Could you check a few things on this model? Use its own coordinates, in mm. Coordinates: 2 decimals unless noted, no trailing zeros. Loops run counter-clockwise (first coordinate to the right, second up) from the corner with the lowest first, then second, coordinate; pieces in that order, holes last.
1) If I drill on line 1 along Y through (x, z) = (139.7, 2.8); line 2 along X through (y, z) = (96, 3.75), over which ranges is the centre line in solid material (lowest first)?
2) Imagine slicing it at B-B on z = 0.9. Give the number of separate pieces and of enclosed holes in the cut face, plus the area to 3 significant figures.
3) Imagine slicing it at A-A on x = 444.5. Please give me the cut outline in (y, z).
4) Thinking about a two-plate mould opening in X: for faces 1 (the face through (161.32, 25.68, 2.35)), 2 (the face through (237, 67, 0)), which applies, released by +X, released by -X, zero draft, split by the parting line, or undercut?
5) Will this pin go through, and if not, where does the flat tip stop? P1, Ø8.5, axis at x = 215.9, y = 28.58, coming from the -Z side.
```python
from build123d import *

# Parameters (mm, degrees)
SKETCH1_R           = 4.7625
BOSS_EXTRUDE1_DEPTH = 4.7625


with BuildPart() as part:
    # Sketch1 → Boss-Extrude1 (new body)
    with BuildSketch(Plane.XY):
        with BuildLine():
            Line((0, 98.425), (12.7, 98.425))
            ThreePointArc((12.7, 98.425), (15.875, 95.25), (12.7, 92.075))
            Line((12.7, 92.075), (0, 92.075))
            Line((0, 92.075), (0, 41.275))
            Line((0, 41.275), (12.7, 41.275))
            ThreePointArc((12.7, 41.275), (15.875, 38.1), (12.7, 34.925))
            Line((12.7, 34.925), (0, 34.925))
            Line((0, 34.925), (0, 0))
            Line((0, 0), (480.21875, 0))
            Line((480.21875, 0), (480.21875, 34.925))
            Line((480.21875, 34.925), (467.51875, 34.925))
            ThreePointArc((467.51875, 34.925), (464.34375, 38.1), (467.51875, 41.275))
            Line((467.51875, 41.275), (480.21875, 41.275))
            Line((480.21875, 41.275), (480.21875, 92.075))
            Line((480.21875, 92.075), (467.51875, 92.075))
            ThreePointArc((467.51875, 92.075), (464.34375, 95.25), (467.51875, 98.425))
            Line((467.51875, 98.425), (480.21875, 98.425))
            Line((480.21875, 98.425), (480.21875, 131.7625))
            Line((480.21875, 131.7625), (0, 131.7625))
            Line((0, 131.7625), (0, 98.425))
        make_face()
        with Locations((38.1, 103.82449821)):
            Circle(SKETCH1_R, mode=Mode.SUBTRACT)
        with Locations((38.1, 28.575703441)):
            Circle(SKETCH1_R, mode=Mode.SUBTRACT)
        with Locations((63.5, 103.82449821)):
            Circle(SKETCH1_R, mode=Mode.SUBTRACT)
        with Locations((63.5, 28.575703441)):
            Circle(SKETCH1_R, mode=Mode.SUBTRACT)
        with Locations((88.9, 103.82449821)):
            Circle(SKETCH1_R, mode=Mode.SUBTRACT)
        with Locations((88.9, 28.575703441)):
            Circle(SKETCH1_R, mode=Mode.SUBTRACT)
        with Locations((114.3, 103.82449821)):
            Circle(SKETCH1_R, mode=Mode.SUBTRACT)
        with Locations((114.3, 28.575703441)):
            Circle(SKETCH1_R, mode=Mode.SUBTRACT)
        with Locations((139.7, 103.82449821)):
            Circle(SKETCH1_R, mode=Mode.SUBTRACT)
        with Locations((139.7, 28.575703441)):
            Circle(SKETCH1_R, mode=Mode.SUBTRACT)
        with Locations((165.1, 103.82449821)):
            Circle(SKETCH1_R, mode=Mode.SUBTRACT)
        with Locations((165.1, 28.575703441)):
            Circle(SKETCH1_R, mode=Mode.SUBTRACT)
        with Locations((190.5, 103.82449821)):
            Circle(SKETCH1_R, mode=Mode.SUBTRACT)
        with Locations((190.5, 28.575703441)):
            Circle(SKETCH1_R, mode=Mode.SUBTRACT)
        with Locations((215.9, 103.82449821)):
            Circle(SKETCH1_R, mode=Mode.SUBTRACT)
        with Locations((215.9, 28.575703441)):
            Circle(SKETCH1_R, mode=Mode.SUBTRACT)
        with Locations((241.3, 103.82449821)):
            Circle(SKETCH1_R, mode=Mode.SUBTRACT)
        with Locations((241.3, 28.575703441)):
            Circle(SKETCH1_R, mode=Mode.SUBTRACT)
        with Locations((266.7, 103.82449821)):
            Circle(SKETCH1_R, mode=Mode.SUBTRACT)
        with Locations((266.7, 28.575703441)):
            Circle(SKETCH1_R, mode=Mode.SUBTRACT)
        with Locations((292.1, 103.82449821)):
            Circle(SKETCH1_R, mode=Mode.SUBTRACT)
        with Locations((292.1, 28.575703441)):
            Circle(SKETCH1_R, mode=Mode.SUBTRACT)
        with Locations((317.5, 103.82449821)):
            Circle(SKETCH1_R, mode=Mode.SUBTRACT)
        with Locations((317.5, 28.575703441)):
            Circle(SKETCH1_R, mode=Mode.SUBTRACT)
        with Locations((342.9, 103.82449821)):
            Circle(SKETCH1_R, mode=Mode.SUBTRACT)
        with Locations((342.9, 28.575703441)):
            Circle(SKETCH1_R, mode=Mode.SUBTRACT)
        with Locations((368.3, 103.82449821)):
            Circle(SKETCH1_R, mode=Mode.SUBTRACT)
        with Locations((368.3, 28.575703441)):
            Circle(SKETCH1_R, mode=Mode.SUBTRACT)
        with Locations((393.7, 103.82449821)):
            Circle(SKETCH1_R, mode=Mode.SUBTRACT)
        with Locations((393.7, 28.575703441)):
            Circle(SKETCH1_R, mode=Mode.SUBTRACT)
        with Locations((419.1, 103.82449821)):
            Circle(SKETCH1_R, mode=Mode.SUBTRACT)
        with Locations((419.1, 28.575703441)):
            Circle(SKETCH1_R, mode=Mode.SUBTRACT)
        with Locations((444.5, 103.82449821)):
            Circle(SKETCH1_R, mode=Mode.SUBTRACT)
        with Locations((444.5, 28.575703441)):
            Circle(SKETCH1_R, mode=Mode.SUBTRACT)
    extrude(amount=BOSS_EXTRUDE1_DEPTH)


solid = part.part
```
Filled in:
1. line 1: y = 0 to 23.81, 33.34 to 99.06, 108.59 to 131.76
1. line 2: x = 15.79 to 464.43
2. separate pieces: 1
2. enclosed holes: 34
2. area: 60,500 mm2
3. outline: (0, 0) - (23.81, 0) - (23.81, 4.76) - (0, 4.76) - close; (33.34, 0) - (99.06, 0) - (99.06, 4.76) - (33.34, 4.76) - close; (108.59, 0) - (131.76, 0) - (131.76, 4.76) - (108.59, 4.76) - close
4. face 1: undercut
4. face 2: zero draft
5. P1: passes through
